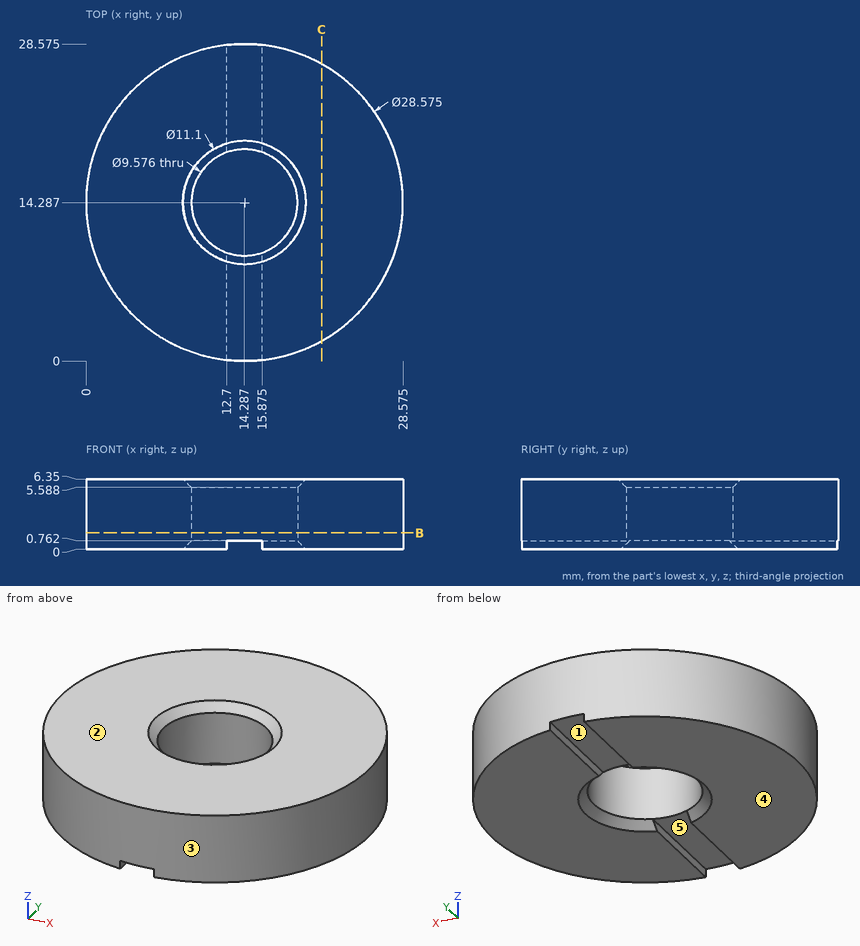
Part print with two shaded views. Sizes in mm from the minimum x, y, z corner. A direction names the side the tool comes from. Give positions to 0.01 mm unless a question says otherwise; leave off trailing zeros. Order: outer loops, then holes, each group sorted by start corner. A loop starts at its lowest first (then second) coordinate and runs counter-clockwise, first axis right, second up. Notation, with made-up numbers: M 59,72 L 79,72 A14 cw 79,87 Z; hole C 1,68.25 d9. An arc over 180 degrees is marked long. Put each result on its own line as item: value.
Item 1: Cut at C-C on x = 21.25. Write the cut outline in (y, z).
Results are:
outline: M 1.81,0 L 26.76,0 L 26.76,6.35 L 1.81,6.35 Z
Item 2: Drop flat-ended pins along their axis: pin 1 Ø8.5 at (x, y) = (14.29, 14.29) entering from -Z (3 decimals); pin 2 Ø3 at (x, z) = (24, 2) entering from -Y (1 decimal); pin 3 Ø0.8 at (y, z) = (26, 0.5) entering from +X (1 decimal); pin 4 Ø1 at (x, z) = (9, 1.5) entering from -Y (1 decimal). Give the stop position or say it passes through.
Results are:
pin 1: through
pin 2: y = 2.6
pin 3: x = 23
pin 4: y = 0.8
Item 3: Wall check: probe 1 along Z at (x, y) = (14, 22); probe 2 along X at (y, z) = (12.5, 3.75) (1 decimal); probe 3 along Y at (x, z) = (15.75, 4.5) (1 decimal). Give the ranges that are in metal, low to high.
Results are:
probe 1: 0.76 to 6.35
probe 2: 0.1 to 9.8, 18.7 to 28.5
probe 3: 0.1 to 9.7, 18.8 to 28.5
Item 4: Which spindle directions (+Z, -Z, +X, -X, +Y, -Y) get a long thin tool onto all of the face, cutting with end or side? Do the marked faces 1 and 2. Say none if no direction does.
Results are:
face 1: -Z, +Y, -Y
face 2: +Z, +X, -X, +Y, -Y
Item 5: Pull direction X, two halves, no side cores. Call the marked faces 3, 4 and 5: +X half, -X half, draft (parallel to the pull), parting line (faces both ways), or undercut.
Results are:
face 3: parting line
face 4: draft
face 5: undercut
Item 6: Cut at B-B on z = 1.5. Write the cut outline in (x, y) (1 decimal), then the cut area to 3 significant figures.
Results are:
outline: C 14.3,14.3 d28.6; hole C 14.3,14.3 d9.6
area: 569 mm2
